```python
from build123d import *

# Parameters (mm, degrees)
F1_DEPTH = 14.224
F0_W     = 6.35
F0_H     = 28.448
F2_DEPTH = 7.874
F3_DEPTH = 7.874
F4_DEPTH = 12.7
F5_W     = 4.7752308284
F5_H     = 28.448
F6_DEPTH = 4.572
F5_W_2   = 7.701497525
F5_H_2   = 30.8059919626
F7_DEPTH = 4.318


with BuildPart() as f1:
    # F0 (on Front) → F1 (new body, symmetric)
    with BuildSketch(Plane.XZ):
        Polygon((-41.7818096255, 18.2387964344), (-48.1318096255, 18.2387964344), (-48.1318096255, -13.7652035656), (-41.7818096255, -13.7652035656), (24.7846730053, -13.7652035656), (24.7846730053, 18.2387964344), align=None)
    extrude(amount=F1_DEPTH, both=True)

    # F0 (on Front) → F2 (join, symmetric)
    with BuildSketch(Plane.XZ):
        Polygon((24.7846730053, -13.7652035656), (-41.7818096255, -13.7652035656), (-41.7818096255, -42.2132035656), (31.1161903745, -42.2132035656), (31.1161903745, -25.1952035656), (39.4981903745, -25.1952035656), (28.0681903745, -13.7652035656), align=None)
        with BuildLine():
            ThreePointArc((-17.5326519589, -33.5772035656), (-23.4938096255, -27.9892035656), (-17.5326519589, -22.4012035656))
            Line((-17.5326519589, -22.4012035656), (16.7847272865, -22.4012035656))
            ThreePointArc((16.7847272865, -22.4012035656), (17.1586896227, -22.3887043175), (17.5326519589, -22.4012035656))
            ThreePointArc((17.5326519589, -22.4012035656), (22.7591888709, -27.9892035656), (17.5326519589, -33.5772035656))
            ThreePointArc((17.5326519589, -33.5772035656), (17.1586896227, -33.5897028138), (16.7847272865, -33.5772035656))
            Line((16.7847272865, -33.5772035656), (-17.5326519589, -33.5772035656))
        make_face(mode=Mode.SUBTRACT)
        Polygon((30.988478276, 46.6867964344), (-41.7818096255, 46.6867964344), (-41.7818096255, 18.2387964344), (24.7846730053, 18.2387964344), (28.0681903745, 18.2387964344), (39.4986695909, 29.6692756508), (30.988478276, 29.6692756508), align=None)
        with BuildLine():
            ThreePointArc((17.526, 38.0507964344), (22.7502411118, 32.4627964344), (17.526, 26.8747964344))
            ThreePointArc((17.526, 26.8747964344), (17.1495770209, 26.8621323434), (16.7731540417, 26.8747964344))
            Line((16.7731540417, 26.8747964344), (-17.526, 26.8747964344))
            ThreePointArc((-17.526, 26.8747964344), (-23.50308707, 32.4627964344), (-17.526, 38.0507964344))
            Line((-17.526, 38.0507964344), (16.7731540417, 38.0507964344))
            ThreePointArc((16.7731540417, 38.0507964344), (17.1495770209, 38.0634605253), (17.526, 38.0507964344))
        make_face(mode=Mode.SUBTRACT)
        with Locations((-44.9568096255, 32.4627964344)):
            Rectangle(F0_W, F0_H)
        with Locations((-44.9568096255, -27.9892035656)):
            Rectangle(F0_W, F0_H)
    extrude(amount=F2_DEPTH, both=True)

    # F0 (on Front) → F3 (join, symmetric)
    with BuildSketch(Plane.XZ):
        Polygon((30.988478276, 46.6867964344), (-41.7818096255, 46.6867964344), (-41.7818096255, 18.2387964344), (24.7846730053, 18.2387964344), (28.0681903745, 18.2387964344), (39.4986695909, 29.6692756508), (30.988478276, 29.6692756508), align=None)
        with BuildLine():
            ThreePointArc((17.526, 38.0507964344), (22.7502411118, 32.4627964344), (17.526, 26.8747964344))
            ThreePointArc((17.526, 26.8747964344), (17.1495770209, 26.8621323434), (16.7731540417, 26.8747964344))
            Line((16.7731540417, 26.8747964344), (-17.526, 26.8747964344))
            ThreePointArc((-17.526, 26.8747964344), (-23.50308707, 32.4627964344), (-17.526, 38.0507964344))
            Line((-17.526, 38.0507964344), (16.7731540417, 38.0507964344))
            ThreePointArc((16.7731540417, 38.0507964344), (17.1495770209, 38.0634605253), (17.526, 38.0507964344))
        make_face(mode=Mode.SUBTRACT)
        with Locations((-44.9568096255, 32.4627964344)):
            Rectangle(F0_W, F0_H)
        with Locations((-44.9568096255, -27.9892035656)):
            Rectangle(F0_W, F0_H)
        Polygon((24.7846730053, -13.7652035656), (-41.7818096255, -13.7652035656), (-41.7818096255, -42.2132035656), (31.1161903745, -42.2132035656), (31.1161903745, -25.1952035656), (39.4981903745, -25.1952035656), (28.0681903745, -13.7652035656), align=None)
        with BuildLine():
            ThreePointArc((-17.5326519589, -33.5772035656), (-23.4938096255, -27.9892035656), (-17.5326519589, -22.4012035656))
            Line((-17.5326519589, -22.4012035656), (16.7847272865, -22.4012035656))
            ThreePointArc((16.7847272865, -22.4012035656), (17.1586896227, -22.3887043175), (17.5326519589, -22.4012035656))
            ThreePointArc((17.5326519589, -22.4012035656), (22.7591888709, -27.9892035656), (17.5326519589, -33.5772035656))
            ThreePointArc((17.5326519589, -33.5772035656), (17.1586896227, -33.5897028138), (16.7847272865, -33.5772035656))
            Line((16.7847272865, -33.5772035656), (-17.5326519589, -33.5772035656))
        make_face(mode=Mode.SUBTRACT)
    extrude(amount=F3_DEPTH, both=True)

    # F0 (on Front) → F4 (join, symmetric)
    with BuildSketch(Plane.XZ):
        Polygon((56.5161903745, 46.6867964344), (30.988478276, 46.6867964344), (30.988478276, 29.6692756508), (39.4986695909, 29.6692756508), align=None)
        Polygon((31.1161903745, -25.1952035656), (31.1161903745, -42.2132035656), (56.5161903745, -42.2132035656), (39.4981903745, -25.1952035656), align=None)
    extrude(amount=F4_DEPTH, both=True)

    # F5 (on face) → F6 (cut, symmetric)
    with BuildSketch(Plane.XZ.offset(7.874)):
        with Locations((-45.7441942113, 32.4627964344)):
            Rectangle(F5_W, F5_H)
    extrude(amount=F6_DEPTH, both=True, mode=Mode.SUBTRACT)

    # F5 (on face) → F7 (cut, symmetric)
    with BuildSketch(Plane.XZ.offset(7.874)):
        with Locations((-47.2073275596, -29.8076486215)):
            Rectangle(F5_W_2, F5_H_2)
        with Locations((-45.7441942113, 32.4627964344)):
            Rectangle(F5_W, F5_H)
    extrude(amount=F7_DEPTH, both=True, mode=Mode.SUBTRACT)


solid = f1.part
```
Source: CAD feature listing. Evaluate the final solid. Frame: model axes, mm. A direction names the side the tool comes from. Round coordinates to 2 decimals unless told otherwise and drop trailing zeros. Loops run counter-clockwise (first coordinate to the right, second up) from the corner with the lowest first, then second, coordinate; pieces in that order, holes last. Notation, with made-up numbers: M 70,39 L 122,39 A29 cw 122,64 Z; hole C -10,74 d3. An arc over 180 degrees is marked long. Use a Markdown table: item, result. Add a question column.
1. Pull-direction query (X, two-part tool) for faces 5 (the flat face through (41, 12.7, -35)), 6 (the flat face through (30.988, -10, 38)), 7 (the cylindrical face through (-23.5, -0.1, 32.3)), 8 (the flat face through (-1, 0, -22.401)); classes: +X half, -X half, draft (parallel to the pull), parting line (faces both ways), or undercut.
2. Cut plane D-D, the plane z = -19. Output: boundary loops of the cut face in (x, y).
3. Set-up query: faces 1 (the flat face through (31.116, 10, -34)), 2 (the flat face through (-43.357, -6, -29)), 3 (the flat face through (35, 10, 29.669)), 4 (the flat face through (35, -10, 29.669)). Return all of +Z, -Z, +X, -X, +Y, -Y with unobstructed straight access to the full face (end or side cutting, diameter ignored); none if empty.
4. Cut plane B-B, the plane x = -26. Output: boundary loops of the cut face in (y, z), and give its area (3 significant figures).
5. Contact query for flat-ended pins moving along their axis: pin 1 (6 mm diameter, centred on y = 7.5, z = 25, fed in from +X); pin 2 (18.5 mm diameter, centred on x = 43, z = 37, fed in from -Y); pin 3 (4 mm diameter, centred on x = -45, z = 31.5, fed in from -Y). Output: stop coordinate, or through.
6. Ray query, line 1 along Z through (x, y) = (4, 6.25); line 2 along Z through (x, y) = (34, 9.25); line 3 along X through (y, z) = (8, 3). Return the intervals inside material, ascending. Write a range as [from, to].
7. Cut plane A-A, the plane x = -4. Output: boundary loops of the cut face in (y, z).
8. Cut plane C-C, the plane x = 49. Output: boundary loops of the cut face in (y, z), and give its area (3 significant figures).
Solution:
| question | item | result |
|---|---|---|
| 1 | face 5 | draft |
| 1 | face 6 | -X half |
| 1 | face 7 | undercut |
| 1 | face 8 | undercut |
| 2 | outline | M -48.13,-3.56 L -43.36,-3.56 L -43.36,-7.87 L 33.3,-7.87 L 33.3,7.87 L -48.13,7.87 Z |
| 3 | face 1 | -Z, -X, +Y |
| 3 | face 2 | -Z, -X, -Y |
| 3 | face 3 | +X, -X, +Y |
| 3 | face 4 | +X, -X, -Y |
| 4 | outline | M -14.22,-13.77 L -7.87,-13.77 L -7.87,-42.21 L 7.87,-42.21 L 7.87,-13.77 L 14.22,-13.77 L 14.22,18.24 L 7.87,18.24 L 7.87,46.69 L -7.87,46.69 L -7.87,18.24 L -14.22,18.24 Z |
| 4 | area | 1,810 mm2 |
| 5 | pin 1 | stops at x = 37.83 |
| 5 | pin 2 | stops at y = -12.7 |
| 5 | pin 3 | stops at y = -7.87 |
| 6 | line 1 | z = [-42.21, -33.58], [-22.4, 26.87], [38.05, 46.69] |
| 6 | line 2 | z = [-42.21, -25.2], [29.67, 46.69] |
| 6 | line 3 | x = [-48.13, 24.78] |
| 7 | outline | M -14.22,-13.77 L -7.87,-13.77 L -7.87,-22.4 L 7.87,-22.4 L 7.87,-13.77 L 14.22,-13.77 L 14.22,18.24 L 7.87,18.24 L 7.87,26.87 L -7.87,26.87 L -7.87,18.24 L -14.22,18.24 Z; M -7.87,-42.21 L 7.87,-42.21 L 7.87,-33.58 L -7.87,-33.58 Z; M -7.87,38.05 L 7.87,38.05 L 7.87,46.69 L -7.87,46.69 Z |
| 8 | outline | M -12.7,-42.21 L 12.7,-42.21 L 12.7,-34.7 L -12.7,-34.7 Z; M -12.7,39.17 L 12.7,39.17 L 12.7,46.69 L -12.7,46.69 Z |
| 8 | area | 382 mm2 |
